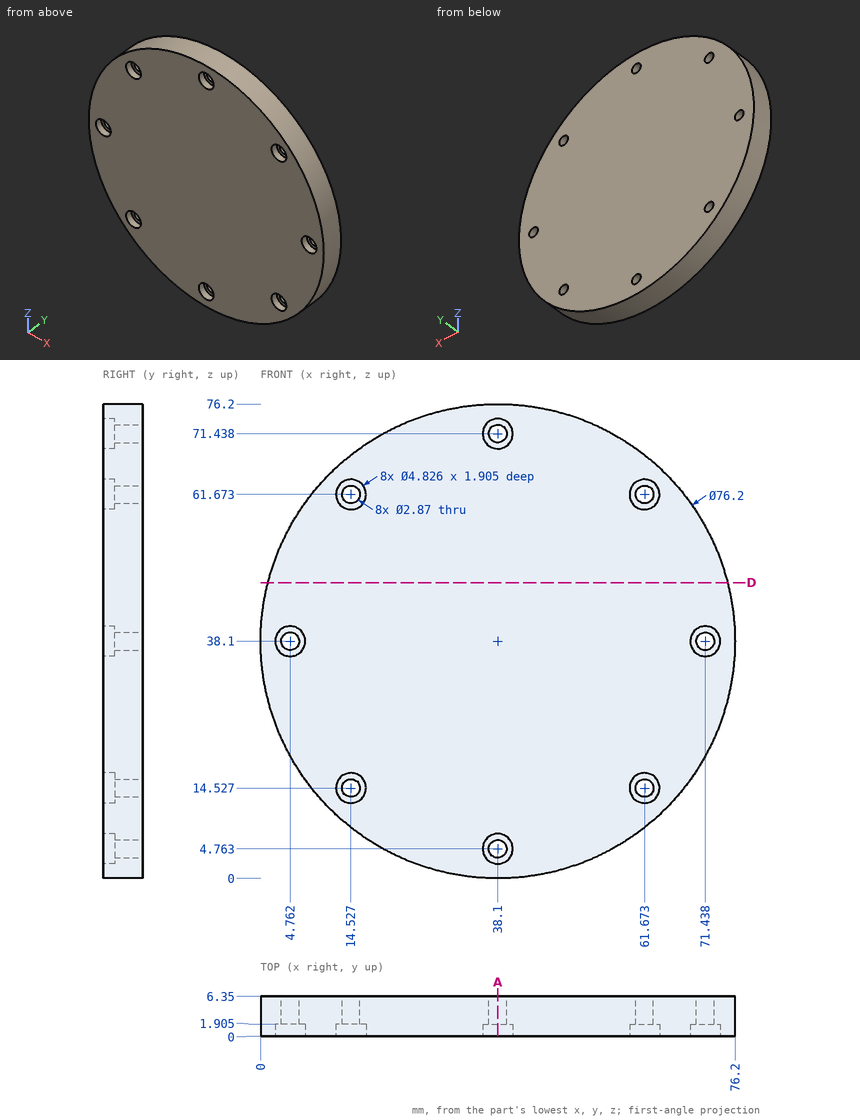
Verification items for this drawing (mm, ordinates from the low corner). Round coordinates to 2 decimals unless told otherwise and drop trailing zeros. Write each loop counter-clockwise with the first axis right and the second up, starting at its lowest first coordinate (ties: lowest second). Pieces come first, ordered by that corner, then holes. Notation, with made-up numbers: (-33, 66) - (22, 66) arc R23 ccw to (22, 90) - close; hole circle Ø3 at (21, 26.5). An arc over 180 degrees is marked (long way). Answer as a JSON object with one key per item and string values. Group by question number.
Q1. Section check D-D, the plane z = 47.5. Enter the section's corners in (x, y), plus the area to 3 significant figures.
Q2. Section check A-A, the plane x = 38.1. Give the number of separate pieces and of enclosed holes in the cut face, plus the area to 3 significant figures.
Q3. Thickness scan on line 1 (Z direction, x = 38, y = 5) (1 decimal); line 2 (X direction, y = 1.5, z = 60.5) (1 decimal); line 3 (X direction, y = 5, z = 5) (1 decimal). Record the ranges inside material, lowest first.
Q4. Go/stop test with flat-tipped pins: pin 1 Ø2.5 at (x, z) = (61.5, 13.5) entering from -Y (1 decimal); pin 2 Ø1.5 at (x, y) = (66.5, 4.5) entering from +Z; pin 3 Ø5.5 at (x, z) = (61.67, 61.67) entering from +Y; pin 4 Ø2 at (y, z) = (3, 11.5) entering from +X. Record where each tip stops, or that it passes through.
Found:
{
 "1": {"outline": "(1.18, 0) - (75.02, 0) - (75.02, 6.35) - (1.18, 6.35) - close", "area": "469 mm^2"},
 "2": {"separate pieces": "3", "enclosed holes": "0", "area": "440 mm^2"},
 "3": {"line 1": "z = 0 to 3.3, 6.2 to 70, 72.9 to 76.2", "line 2": "x = 7.3 to 12.4, 16.6 to 59.6, 63.8 to 68.9", "line 3": "x = 19.2 to 36.7, 39.5 to 57"},
 "4": {"pin 1": "stops at y = 1.9", "pin 2": "stops at z = 64.31", "pin 3": "stops at y = 6.35", "pin 4": "stops at x = 66.32"}
}
